```python
from build123d import *

# Parameters (mm, degrees)
F1_DEPTH = 63.5
F2_DEPTH = 25.4
F0_W     = 25.4
F0_H     = 19.05
F3_DEPTH = 25.4
F4_DEPTH = 7.9375
F6_R     = 6.35


with BuildPart() as f1:
    # F0 (on Front) → F1 (new body, symmetric)
    with BuildSketch(Plane.XZ):
        Polygon((-41.275, 9.525), (-41.275, -9.525), (41.275, -9.525), (41.275, 9.525), (22.225, 9.525), align=None)
    extrude(amount=F1_DEPTH, both=True)

    # F0 (on Front) → F2 (join, symmetric)
    with BuildSketch(Plane.XZ):
        with BuildLine():
            Line((22.225, 9.525), (41.275, 9.525))
            Line((41.275, 9.525), (41.275, 27.0002))
            ThreePointArc((41.275, 27.0002), (45.9246798487, 38.2255201513), (57.15, 42.8752))
            Line((57.15, 42.8752), (60.325, 42.8752))
            Line((60.325, 42.8752), (60.325, 61.9252))
            Line((60.325, 61.9252), (57.15, 61.9252))
            add(Edge.make_bspline(
                [(53.6196332625, 61.7463096484), (54.8063742239, 61.8190464484), (55.9836636447, 61.878690137), (57.15, 61.9252)],
                knots=[108.3511799564, 108.3511799564, 108.3511799564, 108.3511799564, 111.5045361635, 111.5045361635, 111.5045361635, 111.5045361635], degree=3))
            ThreePointArc((53.6196332625, 61.7463096484), (31.2361650531, 50.4144858816), (22.225, 27.0002))
            Line((22.225, 27.0002), (22.225, 9.525))
        make_face()
    extrude(amount=F2_DEPTH, both=True)

    # F0 (on Front) → F3 (join, symmetric)
    with BuildSketch(Plane.XZ):
        with Locations((73.025, 52.4002)):
            Rectangle(F0_W, F0_H)
    extrude(amount=F3_DEPTH, both=True)

    # F0 (on Front) → F4 (join, symmetric)
    with BuildSketch(Plane.XZ):
        with BuildLine():
            add(Edge.make_bspline(
                [(-41.275, 9.525), (-39.0935689496, 41.2893669107), (12.8425135763, 59.2470302808), (53.6196332625, 61.7463096484)],
                knots=[0, 0, 0, 0, 108.3511799564, 108.3511799564, 108.3511799564, 108.3511799564], degree=3))
            Line((-41.275, 9.525), (22.225, 9.525))
            Line((22.225, 9.525), (22.225, 27.0002))
            ThreePointArc((22.225, 27.0002), (31.2361650531, 50.4144858816), (53.6196332625, 61.7463096484))
        make_face()
    extrude(amount=F4_DEPTH, both=True)

    # F0 (on Front) → F5 (revolve)
    with BuildSketch(Plane.XZ):
        Polygon((85.725, 66.675), (85.725, 61.9252), (85.725, 42.8752), (85.725, 38.1), (111.125, 38.1), (111.125, 66.675), align=None)
    revolve(axis=Axis((85.725, 0, 52.3875), (0, 0, 1)))

    # F6
    f6_edges = [f1.edges().sort_by_distance(p)[0] for p in [
        (41.275, -63.5, 0),
        (41.275, 63.5, 0),
        (-41.275, -63.5, 0),
        (-41.275, 63.5, 0),
    ]]
    fillet(f6_edges, radius=F6_R)


solid = f1.part
```
The model under review builds one solid part; all positions refer to its coordinate system, in mm. A direction names the side the tool comes from. Round coordinates to 2 decimals unless told otherwise and drop trailing zeros. Write each loop counter-clockwise with the first axis right and the second up, starting at its lowest first coordinate (ties: lowest second). Pieces come first, ordered by that corner, then holes.
(1) Mouldability with a two-part tool opening along X and no side actions: class faces 5 (the flat face through (41.275, -1, 4)), 6 (the flat face through (60, 2, 42.875)), 7 (the flat face through (-4, 7.938, 30)) as +X half, -X half, draft (parallel to the pull), parting line (faces both ways), or undercut.
(2) Insertion check: pin 1 (2 mm diameter, centred on y = -14.5, z = 43, fed in from +X); pin 2 (1 mm diameter, centred on y = -1, z = 20, fed in from -X); pin 3 (5 mm diameter, centred on y = -14, z = 17.5, fed in from -X) (3 decimals). Each pin has a flat end and moves straight along its axis. Give the tip position at first contact, or say it passes through.
(3) We need section C-C on x = 99. Give the boundary of the cut face in (y, z) (3 decimals).
(4) Wall thickness on L1, parallel to Z at x = 95.5, y = -20 (3 decimals); L2, parallel to X at y = 31.5, z = 5 (3 decimals); L3, parallel to Z at x = 16.5, y = -20.5 (3 decimals): over which ranges is each line inside the solid? List them lowest first.
(5) Machinability: for faces 1 (the flat face through (86, 0, 38.1)), 2 (the flat face through (46, -25.4, 42)), 3 (the flat face through (22.225, -17, 18)), 4 (the cylindrical face through (45.8, -0.4, 38.1)), which of the approach directions +Z, -Z, +X, -X, +Y, -Y give a long, thin tool a straight path to every point of the face, cutting with its end or side? Answer none if there is none.
(6) We need section B-B on y = -35. Give the boundary of the cut face in (x, z) (3 decimals), and give its area (3 significant figures).
(7) We need section A-A on z = -2. Give the boundary of the cut face in (x, y) (3 decimals).
Findings below:
1. face 5: +X half
1. face 6: undercut
1. face 7: draft
2. pin 1: stops at x = 107.24
2. pin 2: stops at x = -38.83
2. pin 3: stops at x = 22.225
3. outline: (-21.655, 38.1) - (21.655, 38.1) - (21.655, 66.675) - (-21.655, 66.675) - close
4. L1: z = 38.1 to 66.675
4. L2: x = -41.275 to 41.275
4. L3: z = -9.525 to 9.525
5. face 1: -Z, +X, +Y, -Y
5. face 2: +Z, +X, -X, -Y
5. face 3: +Z, -X, -Y
5. face 4: -Z, +Y, -Y
6. outline: (-41.275, -9.525) - (41.275, -9.525) - (41.275, 9.525) - (-41.275, 9.525) - close
6. area: 1,570 mm2
7. outline: (-41.275, -57.15) arc R6.35 ccw to (-34.925, -63.5) - (34.925, -63.5) arc R6.35 ccw to (41.275, -57.15) - (41.275, 57.15) arc R6.35 ccw to (34.925, 63.5) - (-34.925, 63.5) arc R6.35 ccw to (-41.275, 57.15) - close
